from build123d import *

# Parameters (mm, degrees)
F0_W     = 609.6
F0_H     = 914.4
F1_DEPTH = 19.05
F2_W     = 101.6
F2_H     = 279.4
F3_DEPTH = 3.175
F4_W     = 88.9
F4_H     = 266.7
F5_DEPTH = 25.4


with BuildPart() as f1:
    # F0 (on Top) → F1 (new body)
    with BuildSketch(Plane.XY):
        Rectangle(F0_W, F0_H)
    extrude(amount=F1_DEPTH)

    # F2 (on face) → F3 (cut)
    with BuildSketch(Plane.XY.offset(19.05)):
        with Locations((12.7, 0)):
            Rectangle(F2_W, F2_H)
    extrude(amount=-F3_DEPTH, mode=Mode.SUBTRACT)

    # F4 (on face) → F5 (cut)
    with BuildSketch(Plane.XY.offset(15.875)):
        with Locations((12.7, 0)):
            Rectangle(F4_W, F4_H)
    extrude(amount=-F5_DEPTH, mode=Mode.SUBTRACT)


solid = f1.part
Geometry: final body of the model. Coordinates: model frame, mm. A direction names the side the tool comes from. Give positions to 0.01 mm unless a question says otherwise; leave off trailing zeros. Write each loop counter-clockwise with the first axis right and the second up, starting at its lowest first coordinate (ties: lowest second). Pieces come first, ordered by that corner, then holes.
(1) Cut plane B-B, the plane z = 10.5. Return loops of the section in (x, y), then the cut area to 3 significant figures.
(2) Cut plane A-A, the plane x = 4. Return loops of the section in (y, z) (3 decimals).
(3) Cut plane C-C, the plane y = 37.5. Return loops of the section in (x, z) (3 decimals).
(4) First-contact query: P1, Ø10, axis at x = 75, y = -276, coming from the -Z side. Flat tip, straight axial feed; report the tip coordinate or a pass-through.
(5) Access query for faces 1 (the flat face through (-33, 11, 15.875)), 2 (the flat face through (304.8, -6, 9)). Directions: +Z, -Z, +X, -X, +Y, -Y. A direction counts if a zero-diameter tool reaches every point of the face in a straight line with its end or side. Return the directions, or none.
(6) Ray query, line 1 (Y direction, x = 28.5, z = 11.25); line 2 (Y direction, x = 43, z = 16.75); line 3 (X direction, y = 4, z = 3.5). Return the intervals inside material, ascending.
Values follow:
1. outline: (-304.8, -457.2) - (304.8, -457.2) - (304.8, 457.2) - (-304.8, 457.2) - close; hole (-31.75, -133.35) - (57.15, -133.35) - (57.15, 133.35) - (-31.75, 133.35) - close
1. area: 534,000 mm2
2. outline: (-457.2, 0) - (-133.35, 0) - (-133.35, 15.875) - (-139.7, 15.875) - (-139.7, 19.05) - (-457.2, 19.05) - close; (133.35, 0) - (457.2, 0) - (457.2, 19.05) - (139.7, 19.05) - (139.7, 15.875) - (133.35, 15.875) - close
3. outline: (-304.8, 0) - (-31.75, 0) - (-31.75, 15.875) - (-38.1, 15.875) - (-38.1, 19.05) - (-304.8, 19.05) - close; (57.15, 0) - (304.8, 0) - (304.8, 19.05) - (63.5, 19.05) - (63.5, 15.875) - (57.15, 15.875) - close
4. P1: stops at z = 0
5. face 1: +Z
5. face 2: +Z, -Z, +X, +Y, -Y
6. line 1: y = -457.2 to -133.35, 133.35 to 457.2
6. line 2: y = -457.2 to -139.7, 139.7 to 457.2
6. line 3: x = -304.8 to -31.75, 57.15 to 304.8
